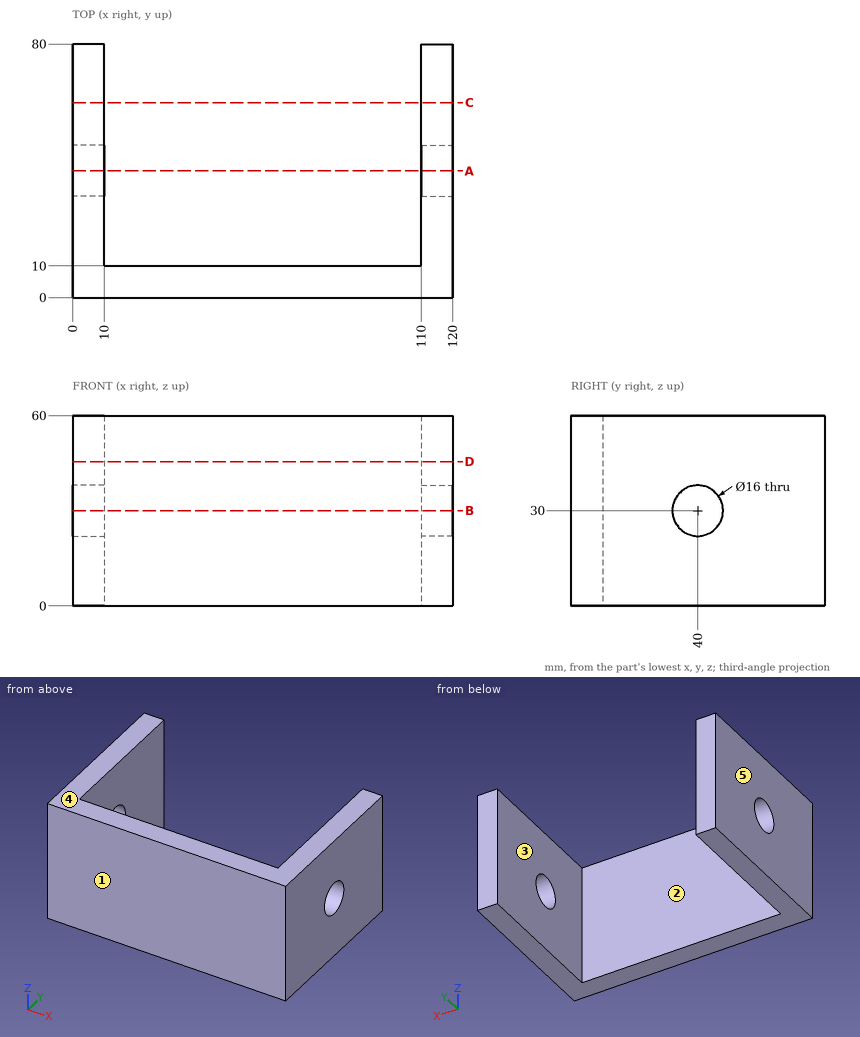
Geometry check sheet. Reference: drawing and pictorial views, mm from the part's lowest x, y, z. A direction names the side the tool comes from. Coordinates: 2 decimals unless noted, no trailing zeros. Loops run counter-clockwise (first coordinate to the right, second up) from the corner with the lowest first, then second, coordinate; pieces in that order, holes last. Notation, with made-up numbers: (-29, 69.5) - (-15, 69.5) arc R20 ccw to (-15, 100.5) - close; hole circle Ø11 at (-10.5, 57.25). An arc over 180 degrees is marked (long way). Return JSON: item names as keys, results as strings.
1. Tool access check on the marked faces 1 and 2. Record the directions out of +Z, -Z, +X, -X, +Y, -Y that give a thin tool (end or side, any length) a straight path to the whole face; none if there is none.
Established:
{"face 1": "+Z, -Z, +X, -X, -Y", "face 2": "+Z, -Z, +Y"}
2. Section check A-A, the plane y = 40. Record the boundary of the cut face in (x, z).
Established:
{"outline": "(0, 0) - (10, 0) - (10, 22) - (0, 22) - close; (0, 38) - (10, 38) - (10, 60) - (0, 60) - close; (110, 0) - (120, 0) - (120, 22) - (110, 22) - close; (110, 38) - (120, 38) - (120, 60) - (110, 60) - close"}
3. Thickness scan on L1, parallel to X at y = 53, z = 17.5; L2, parallel to Y at x = 112, z = 30; L3, parallel to Y at x = 106, z = 31.5. Record the ranges inside material, lowest first.
Established:
{"L1": "x = 0 to 10, 110 to 120", "L2": "y = 0 to 32, 48 to 80", "L3": "y = 0 to 10"}
4. Go/stop test with a flat-tipped pin: pin 1 (5 mm diameter, centred on x = 47, z = 49.5, fed in from +Y). Record where the tip stops, or that it passes through.
Established:
{"pin 1": "stops at y = 10"}
5. Mould release check, pull along X, two halves, no side actions. Record for the marked faces 3, 4 and 5: +X half, -X half, draft (parallel to the pull), parting line (faces both ways), or undercut.
Established:
{"face 3": "undercut", "face 4": "draft", "face 5": "-X half"}
6. Section check C-C, the plane y = 61.5. Record the boundary of the cut face in (x, z), then the cut area to 3 significant figures.
Established:
{"outline": "(0, 0) - (10, 0) - (10, 60) - (0, 60) - close; (110, 0) - (120, 0) - (120, 60) - (110, 60) - close", "area": "1,200 mm2"}
7. Section check D-D, the plane z = 45.5. Record the boundary of the cut face in (x, y).
Established:
{"outline": "(0, 0) - (120, 0) - (120, 80) - (110, 80) - (110, 10) - (10, 10) - (10, 80) - (0, 80) - close"}
8. Section check B-B, the plane z = 30. Record the boundary of the cut face in (x, y).
Established:
{"outline": "(0, 0) - (120, 0) - (120, 32) - (110, 32) - (110, 10) - (10, 10) - (10, 32) - (0, 32) - close; (0, 48) - (10, 48) - (10, 80) - (0, 80) - close; (110, 48) - (120, 48) - (120, 80) - (110, 80) - close"}
